Geometry: final body of the model. Coordinates: model frame, mm. Face numbers are marked on the shaded views. Give positions to 0.01 mm unless a question says otherwise; leave off trailing zeros. Loops run counter-clockwise (first coordinate to the right, second up) from the corner with the lowest first, then second, coordinate; pieces in that order, holes last. Notation, with made-up numbers: M 65.5,88 L 76.5,88 A29 cw 76.5,111 Z; hole C 50.25,-27 d6. An arc over 180 degrees is marked long. One line per question, with ' | ' between items. Start each with the question number.
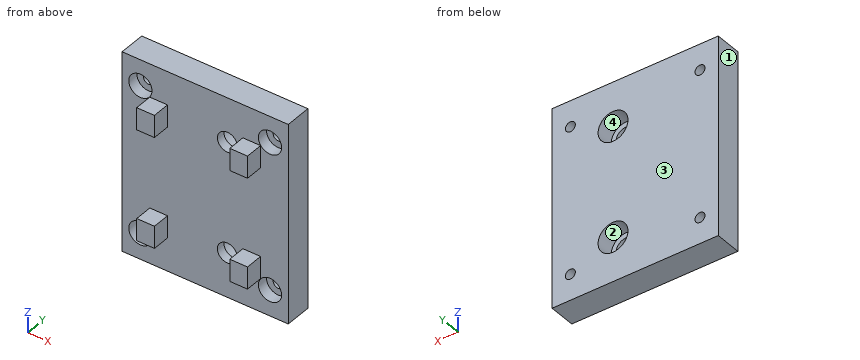
Autodesk Fusion 360 part; units mm, degrees
sketch "Sketch1" plane through (0, 0, 0) normal (0, 1, 0) x (1, 0, 0)
  line L0 (29.25, 33.25) -> (-29.25, 33.25)
  line L1 (-29.25, 33.25) -> (-29.25, -33.25)
  line L2 (-29.25, -33.25) -> (29.25, -33.25)
  line L3 (29.25, -33.25) -> (29.25, 33.25)
  line L4 (29.25, 33.25) -> (-29.25, -33.25) construction
  line L5 (-29.25, 33.25) -> (29.25, -33.25) construction
  circle A0 centre (-29.25, -33.25) radius 2.25
  circle A1 centre (29.25, -33.25) radius 2.25
  circle A2 centre (-29.25, 33.25) radius 2.25
  circle A3 centre (29.25, 33.25) radius 2.25
  line L6 (37.5, 45) -> (-37.5, 45)
  line L7 (-37.5, 45) -> (-37.5, -45)
  line L8 (-37.5, -45) -> (37.5, -45)
  line L9 (37.5, -45) -> (37.5, 45)
  line L10 (37.5, 45) -> (-37.5, -45) construction
  line L11 (-37.5, 45) -> (37.5, -45) construction
  dimension "d1" = 58.5
  dimension "d2" = 66.5
  dimension "d3" = 4.5
  dimension "d4" = 4.5
  dimension "d5" = 4.5
  dimension "d6" = 4.5
  dimension "d7" = 75
  dimension "d8" = 90
extrude "Extrude1" add sketch "Sketch1" along normal blind 12 contours L0 L1 L2 L3 A0 A1 A2 A3 | L6 L7 L8 L9
sketch "Sketch2" plane through (0, 0, 0) normal (0, -1, 0) x (1, 0, 0)
  circle A0 centre (29.25, -33.25) radius 2.25
  circle A1 centre (-29.25, 33.25) radius 2.25
  circle A2 centre (-29.25, -33.25) radius 2.25
  circle A3 centre (29.25, 33.25) radius 2.25
  line L0 (37.5, -45) -> (37.5, 45)
  line L1 (37.5, 45) -> (-37.5, 45)
  line L2 (-37.5, 45) -> (-37.5, -45)
  line L3 (-37.5, -45) -> (37.5, -45)
  line L4 (-35, -30) -> (35, -30)
  line L5 (35, -30) -> (35, 30)
  line L6 (35, 30) -> (-35, 30)
  line L7 (-35, 30) -> (-35, -30)
  line L8 (-35, -30) -> (35, 30) construction
  line L9 (35, -30) -> (-35, 30) construction
  line L10 (-25, -20) -> (-17, -20)
  line L11 (-17, -20) -> (-17, -30)
  line L12 (-17, -30) -> (-25, -30)
  line L13 (-25, -30) -> (-25, -20)
  line L14 (25, -20) -> (17, -20)
  line L15 (17, -20) -> (17, -30)
  line L16 (17, -30) -> (25, -30)
  line L17 (25, -30) -> (25, -20)
  line L18 (25, 20) -> (17, 20)
  line L19 (17, 20) -> (17, 30)
  line L20 (17, 30) -> (25, 30)
  line L21 (25, 30) -> (25, 20)
  line L22 (-25, 20) -> (-17, 20)
  line L23 (-17, 20) -> (-17, 30)
  line L24 (-17, 30) -> (-25, 30)
  line L25 (-25, 30) -> (-25, 20)
  circle A4 centre (10, -25) radius 4.5
  circle A5 centre (-10, -25) radius 4.5
  circle A6 centre (10, 25) radius 4.5
  circle A7 centre (-10, 25) radius 4.5
  dimension "d11" = 60
  dimension "d25" = 8
  dimension "d26" = 8
  dimension "d27" = 8
  dimension "d28" = 8
  dimension "d29" = 9
  dimension "d30" = 9
  dimension "d31" = 9
  dimension "d32" = 9
extrude "Extrude2" add sketch "Sketch2" along normal blind 8 contours L4 L10 L11 L12 L13 | L6 L22 L23 L24 L25 | L4 L14 L15 L16 L17 | L6 L18 L19 L20 L21
sketch "Sketch3" plane through (0, 0, 0) normal (0, -1, 0) x (1, 0, 0)
  line L0 (-25, 30) -> (-17, 30)
  line L1 (25, -30) -> (17, -30)
  line L2 (37.5, -45) -> (37.5, 45)
  line L3 (-37.5, 45) -> (-37.5, -45)
  line L4 (-17, 30) -> (-17, 20)
  line L5 (-17, 20) -> (-25, 20)
  line L6 (-25, 20) -> (-25, 30)
  line L7 (17, -30) -> (17, -20)
  line L8 (17, -20) -> (25, -20)
  line L9 (25, -20) -> (25, -30)
  line L10 (25, 30) -> (25, 20)
  line L11 (25, 20) -> (17, 20)
  line L12 (17, 20) -> (17, 30)
  line L13 (17, 30) -> (25, 30)
  line L14 (-25, -30) -> (-25, -20)
  line L15 (-25, -20) -> (-17, -20)
  line L16 (-17, -20) -> (-17, -30)
  line L17 (-17, -30) -> (-25, -30)
  line L18 (37.5, 45) -> (-37.5, 45)
  line L19 (-37.5, -45) -> (37.5, -45)
  circle A0 centre (29.25, 33.25) radius 2.25
  circle A1 centre (29.25, -33.25) radius 2.25
  circle A2 centre (-29.25, 33.25) radius 2.25
  circle A3 centre (-29.25, -33.25) radius 2.25
  circle A4 centre (29.25, -33.25) radius 5.25
  circle A5 centre (-29.25, -33.25) radius 5.25
  circle A6 centre (-29.25, 33.25) radius 5.25
  circle A7 centre (29.25, 33.25) radius 5.25
  dimension "d41" = 10.5
  dimension "d42" = 10.5
  dimension "d43" = 10.5
  dimension "d44" = 10.5
sketch "Sketch4" plane through (0, 0, 0) normal (0, -1, 0) x (1, 0, 0)
  line L0 (-37.5, 45) -> (-37.5, -45)
  line L1 (25, -30) -> (17, -30)
  line L2 (17, 30) -> (25, 30)
  line L3 (-37.5, -45) -> (37.5, -45)
  line L4 (17, -30) -> (17, -20)
  line L5 (17, -20) -> (25, -20)
  line L6 (25, -20) -> (25, -30)
  line L7 (25, 30) -> (25, 20)
  line L8 (25, 20) -> (17, 20)
  line L9 (17, 20) -> (17, 30)
  line L10 (37.5, -45) -> (37.5, 45)
  line L11 (37.5, 45) -> (-37.5, 45)
  line L12 (-17, 30) -> (-17, 20)
  line L13 (-17, 20) -> (-25, 20)
  line L14 (-25, 20) -> (-25, 30)
  line L15 (-25, -30) -> (-25, -20)
  line L16 (-25, -20) -> (-17, -20)
  line L17 (-17, -20) -> (-17, -30)
  line L18 (-17, -30) -> (-25, -30)
  line L19 (-25, 30) -> (-17, 30)
  circle A0 centre (29.25, 33.25) radius 2.25
  circle A1 centre (-29.25, 33.25) radius 2.25
  circle A2 centre (-29.25, -33.25) radius 2.25
  circle A3 centre (29.25, -33.25) radius 2.25
sketch "Sketch5" plane through (0, 12, 0) normal (0, 1, 0) x (-1, 0, 0)
  circle A0 centre (-29.25, 33.25) radius 2.25
  circle A1 centre (-29.25, -33.25) radius 2.25
  circle A2 centre (29.25, 33.25) radius 2.25
  circle A3 centre (29.25, -33.25) radius 2.25
  line L0 (-37.5, 45) -> (-37.5, -45)
  line L1 (-37.5, -45) -> (37.5, -45)
  line L2 (37.5, -45) -> (37.5, 45)
  line L3 (37.5, 45) -> (-37.5, 45)
  circle A4 centre (10, -25) radius 6.75
  circle A5 centre (-10, -25) radius 6.75
  circle A6 centre (10, 25) radius 6.75
  circle A7 centre (-10, 25) radius 6.75
  dimension "d33" = 13.5
  dimension "d34" = 13.5
  dimension "d35" = 13.5
  dimension "d36" = 13.5
extrude "Extrude4" cut sketch "Sketch5" against normal blind 8 contours A5 | A7
extrude "Extrude5" cut sketch "Sketch2" against normal blind 16 contours A4 | A6
extrude "Extrude6" cut sketch "Sketch3" against normal blind 5 contours A4 | A5 | A6 | A7
Q1. Material intervals for L1, parallel to X at y = 2.25, z = -33; L2, parallel to Z at x = -29.25, y = 8.75; L3, parallel to Z at x = 10, y = 2, sorted ascending.
Q2. Section C-C, the plane y = -5. Output: boundary loops of the cut face in (x, z).
Q3. Draft query along X for the marked faces 1, 2, 3 and 4. Return one class per face: released by +X, released by -X, zero draft, split by the parting line, or undercut.
Q4. Section A-A, the plane z = 33.25. Output: boundary loops of the cut face in (x, y), plus the area to 3 significant figures.
Q5. Contact query for flat-ended pins moving along their axis: pin 1 (4 mm diameter, centred on y = -2.5, z = -27, fed in from +X); pin 2 (4 mm diameter, centred on y = -4, z = 24.5, fed in from -X); pin 3 (3 mm diameter, centred on x = 6, z = 10.5, fed in from -Y). Output: stop coordinate, or through.
Q6. Section D-D, the plane x = 22. Output: boundary loops of the cut face in (y, z), plus the area to 3 significant figures.
Q7. Section B-B, the plane x = 10. Output: boundary loops of the cut face in (y, z), plus the area to 3 significant figures.
Model answer:
1) L1: x = -37.5 to -34.49, -24.01 to 24.01, 34.49 to 37.5 | L2: z = -45 to -35.5, -31 to 31, 35.5 to 45 | L3: z = -45 to -29.5, -20.5 to 20.5, 29.5 to 45
2) outline: M -25,-30 L -17,-30 L -17,-20 L -25,-20 Z; M -25,20 L -17,20 L -17,30 L -25,30 Z; M 17,-30 L 25,-30 L 25,-20 L 17,-20 Z; M 17,20 L 25,20 L 25,30 L 17,30 Z
3) face 1: released by -X | face 2: undercut | face 3: zero draft | face 4: undercut
4) outline: M -37.5,0 L -34.5,0 L -34.5,5 L -31.5,5 L -31.5,12 L -37.5,12 Z; M -27,5 L -24,5 L -24,0 L 24,0 L 24,5 L 27,5 L 27,12 L -27,12 Z; M 31.5,5 L 34.5,5 L 34.5,0 L 37.5,0 L 37.5,12 L 31.5,12 Z | area: 732 mm^2
5) pin 1: stops at x = 25 | pin 2: stops at x = -25 | pin 3: stops at y = 0
6) outline: M -8,-30 L 0,-30 L 0,-45 L 12,-45 L 12,45 L 0,45 L 0,30 L -8,30 L -8,20 L 0,20 L 0,-20 L -8,-20 Z | area: 1,240 mm^2
7) outline: M 0,-45 L 12,-45 L 12,-31.75 L 4,-31.75 L 4,-29.5 L 0,-29.5 Z; M 0,-20.5 L 4,-20.5 L 4,-18.25 L 12,-18.25 L 12,18.25 L 4,18.25 L 4,20.5 L 0,20.5 Z; M 0,29.5 L 4,29.5 L 4,31.75 L 12,31.75 L 12,45 L 0,45 Z | area: 792 mm^2
